Build history of the part. All positions in model axes, mm. A direction names the side the tool comes from. Coordinates: 2 decimals unless noted, no trailing zeros. Write each loop counter-clockwise with the first axis right and the second up, starting at its lowest first coordinate (ties: lowest second). Pieces come first, ordered by that corner, then holes.
from build123d import *

# Parameters (mm, degrees)
SKETCH1_R           = 3.5
BOSS_EXTRUDE1_DEPTH = 6
BOSS_EXTRUDE2_DEPTH = 15


with BuildPart() as part:
    # Sketch1 → Boss-Extrude1 (new body)
    with BuildSketch(Plane.XY):
        with BuildLine():
            Line((-7.5, 0), (-7.5, -15))
            Line((-7.5, -15), (7.5, -15))
            Line((7.5, -15), (7.5, 0))
            ThreePointArc((7.5, 0), (0, 7.5), (-7.5, 0))
        make_face()
        Circle(SKETCH1_R, mode=Mode.SUBTRACT)
    extrude(amount=BOSS_EXTRUDE1_DEPTH)

    # Sketch2 → Boss-Extrude2 (add)
    with BuildSketch(Plane(origin=(7.5, 0, 0), x_dir=(0, 0, -1), z_dir=(1, 0, 0))):
        Polygon((-6, -15), (-33, -17.362193915), (-33, -22.362193915), (-3, -19.737534009), (27, -22.362193915), (27, -17.362193915), (0, -15), align=None)
    extrude(amount=-BOSS_EXTRUDE2_DEPTH)


solid = part.part
(1) Slice it at A-A, the plane x = 0. List the corners of the cut face in (y, z), and give its area (3 significant figures).
(2) Slice it at C-C, the plane z = 1. List the corners of the cut face in (x, y), and give its area (3 significant figures).
(3) Probe L1, parallel to Z at x = 3.5, y = -1.5; L2, parallel to X at y = 1.25, z = 1; L3, parallel to Y at x = 0, z = 2.3. List the from-to ranges inside material, lowest first.
(4) Slice it at D-D, the plane y = -10.5. List the corners of the cut face in (x, z).
(5) 3-axis set-ups, long thin cutter, end or side, ignore diameter. For faces 4 (the flat face through (0, -4, 6)), 5 (the flat face through (0, -4, 0)), 6 (the flat face through (0.11, -21.07, 18.21)): which of +Z, -Z, +X, -X, +Y, -Y reach the whole face in a straight line?
(6) Slice it at B-B, the plane x = -4.5. List the corners of the cut face in (y, z), and give its area (3 significant figures).
(7) Two-plate mould, pull along Z, no slides. Class faces 1 (the flat face through (0.11, -21.03, -11.79)), 2 (the cylindrical face through (3.233, -1.341, 2.958)), 3 (the flat face through (0, -20, -27)): pulls with the +Z half, pulls with the -Z half, needs draft (parallel to the pull), parting line crosses it, or undercut.
(8) Flat gauge pins, fed straight in: P1, Ø6, axis at x = 0, y = 4, coming from the +Z side; P2, Ø9, axis at x = 0, y = 0, coming from the -Z side. Where does each tip first touch, or does it go through?
Results:
1. outline: (-22.36, -27) - (-17.36, -27) - (-15, 0) - (-3.5, 0) - (-3.5, 6) - (-15, 6) - (-17.36, 33) - (-22.36, 33) - (-19.74, 3) - close; (3.5, 0) - (7.5, 0) - (7.5, 6) - (3.5, 6) - close
1. area: 392 mm2
2. outline: (-7.5, -19.91) - (7.5, -19.91) - (7.5, 0) arc R7.5 ccw to (-7.5, 0) - close; hole circle Ø7 at (0, 0)
2. area: 349 mm2
3. L1: z = 0 to 6
3. L2: x = -7.4 to -3.27, 3.27 to 7.4
3. L3: y = -19.8 to -3.5, 3.5 to 7.5
4. outline: (-7.5, 0) - (7.5, 0) - (7.5, 6) - (-7.5, 6) - close
5. face 4: +Z, +X, -X, +Y
5. face 5: -Z, +X, -X, +Y
5. face 6: +X, -X, -Y
6. outline: (-22.36, -27) - (-17.36, -27) - (-15, 0) - (6, 0) - (6, 6) - (-15, 6) - (-17.36, 33) - (-22.36, 33) - (-19.74, 3) - close
6. area: 425 mm2
7. face 1: undercut
7. face 2: needs draft
7. face 3: pulls with the -Z half
8. P1: stops at z = 6
8. P2: stops at z = 0
